Part print with two shaded views. Sizes in mm from the minimum x, y, z corner. A direction names the side the tool comes from. Round coordinates to 2 decimals unless told otherwise and drop trailing zeros. Order: outer loops, then holes, each group sorted by start corner. A loop starts at its lowest first (then second) coordinate and runs counter-clockwise, first axis right, second up. Notation, with made-up numbers: (86, -20.75) -> (103, -20.75) arc R14 ccw to (103, 1.25) -> close; hole circle Ø1 at (26.5, 18). An arc over 180 degrees is marked (long way). Put each result on its own line as item: value. Start each with the question number.
Q1. Pull direction X, two halves, no side cores. Call the marked faces 1, 2 and 3: released by +X, released by -X, zero draft, split by the parting line, or undercut.
Q2. Probe L1, parallel to X at y = 6, z = 10.75; L2, parallel to X at y = 25.4, z = 10.25; L3, parallel to Y at x = 38.1, z = 3.5. List the from-to ranges inside material, lowest first.
Q3. Cut at D-D, the plane y = 6. List the corners of the cut face in (x, z).
Q4. Cut at C-C, the plane y = 25.4. List the corners of the cut face in (x, z).
Q5. Flat gauge pins, fed straight in: P1, Ø15, axis at x = 38.1, y = 25.4, coming from the -Z side; P2, Ø1.9, axis at x = 5, y = 16.5, coming from the +Z side. Where does each tip first touch, or does it go through?
Q6. Cut at A-A, the plane x = 38.1. List the corners of the cut face in (y, z).
Q7. Cut at B-B, the plane z = 11.5. List the corners of the cut face in (x, y), and give its area (3 significant figures).
Q8. 3-axis set-ups, long thin cutter, end or side, ignore diameter. For the marked faces 4 and 5: which of +Z, -Z, +X, -X, +Y, -Y reach the whole face in a straight line?
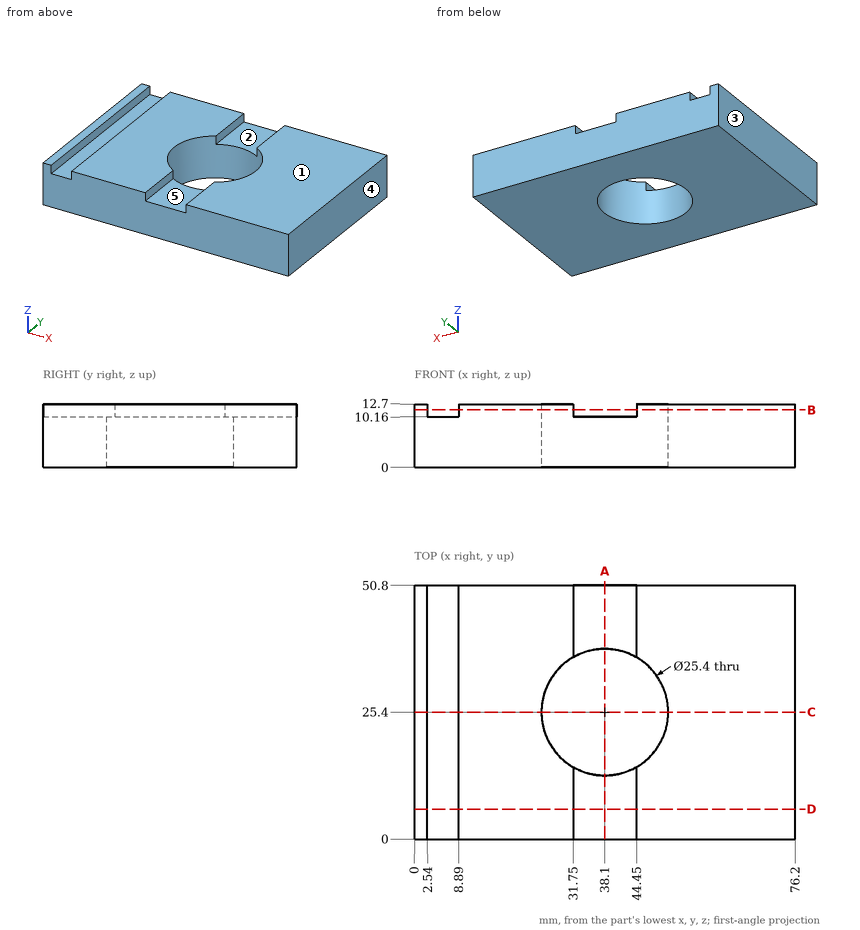
Ans:
1. face 1: zero draft
1. face 2: undercut
1. face 3: released by -X
2. L1: x = 0 to 2.54, 8.89 to 31.75, 44.45 to 76.2
2. L2: x = 0 to 2.54, 8.89 to 25.4, 50.8 to 76.2
2. L3: y = 0 to 12.7, 38.1 to 50.8
3. outline: (0, 0) -> (76.2, 0) -> (76.2, 12.7) -> (44.45, 12.7) -> (44.45, 10.16) -> (31.75, 10.16) -> (31.75, 12.7) -> (8.89, 12.7) -> (8.89, 10.16) -> (2.54, 10.16) -> (2.54, 12.7) -> (0, 12.7) -> close
4. outline: (0, 0) -> (25.4, 0) -> (25.4, 12.7) -> (8.89, 12.7) -> (8.89, 10.16) -> (2.54, 10.16) -> (2.54, 12.7) -> (0, 12.7) -> close; (50.8, 0) -> (76.2, 0) -> (76.2, 12.7) -> (50.8, 12.7) -> close
5. P1: passes through
5. P2: stops at z = 10.16
6. outline: (0, 0) -> (12.7, 0) -> (12.7, 10.16) -> (0, 10.16) -> close; (38.1, 0) -> (50.8, 0) -> (50.8, 10.16) -> (38.1, 10.16) -> close
7. outline: (0, 0) -> (2.54, 0) -> (2.54, 50.8) -> (0, 50.8) -> close; (8.89, 0) -> (31.75, 0) -> (31.75, 14.4) arc R12.7 cw to (31.75, 36.4) -> (31.75, 50.8) -> (8.89, 50.8) -> close; (44.45, 0) -> (76.2, 0) -> (76.2, 50.8) -> (44.45, 50.8) -> (44.45, 36.4) arc R12.7 cw to (44.45, 14.4) -> close
7. area: 2,710 mm^2
8. face 4: +Z, -Z, +X, +Y, -Y
8. face 5: +Z, +Y, -Y
